Model file for the job. Use its own axes, mm. Give positions to 0.01 mm unless a question says otherwise; leave off trailing zeros. Order: outer loops, then holes, each group sorted by start corner. A loop starts at its lowest first (then second) coordinate and runs counter-clockwise, first axis right, second up. Notation, with made-up numbers: (50.25, 66) -> (95.25, 66) arc R8 ccw to (95.25, 70) -> close; hole circle Ø4 at (9, 80). An arc over 180 degrees is marked (long way). Use CSV: the item, a comma, the result in double quotes. Start each with the question number.
1. Cut at B-B on y = 6. List the corners of the cut face in (x, z).
2. Wall check: line 1 (X direction, y = 93, z = 12.5); line 2 (X direction, y = 21, z = -18); line 3 (Y direction, x = 22, z = -18). Give the ranges that are in metal, low to high. Write a range as from..to.
3. Pull direction X, two halves, no side cores. Call faces 1 (the cylindrical face through (142.94, 50.56, 23.72)), 2 (the cylindrical face through (-51.2, 50.56, -20.42)), 3 (the flat face through (45, 0, 1)): released by +X, released by -X, zero draft, split by the parting line, or undercut.
4. Cut at A-A on x = 107. List the corners of the cut face in (y, z).
```python
from build123d import *

# Parameters (mm, degrees)
ESBO_O1_W                = 200
ESBO_O1_H                = 50
RESSALTO_EXTRUS_O1_DEPTH = 100
FILETE9_R                = 10


with BuildPart() as part:
    # Esboço1 → Ressalto-extrusão1 (new body)
    with BuildSketch(Plane(origin=(0, 0, 0), x_dir=(1, 0, 0), z_dir=(0, 1, 0))):
        with Locations((45.947958133, -1.570526198)):
            Rectangle(ESBO_O1_W, ESBO_O1_H)
    extrude(amount=RESSALTO_EXTRUS_O1_DEPTH)

    # Filete9
    filete9_edges = [part.edges().sort_by_distance(p)[0] for p in [
        (145.947958133, 100, 1.570526198),
        (45.947958133, 100, -23.429473802),
        (-54.052041867, 100, 1.570526198),
        (45.947958133, 0, -23.429473802),
        (145.947958133, 0, 1.570526198),
        (45.947958133, 0, 26.570526198),
        (-54.052041867, 0, 1.570526198),
        (45.947958133, 100, 26.570526198),
        (-54.052041867, 50, -23.429473802),
        (145.947958133, 50, -23.429473802),
        (145.947958133, 50, 26.570526198),
        (-54.052041867, 50, 26.570526198),
    ]]
    fillet(filete9_edges, radius=FILETE9_R)


solid = part.part
```
Verdict:
1,outline,"(-53.22, -13.43) arc R9.17 ccw to (-44.05, -22.59) -> (135.95, -22.59) arc R9.17 ccw to (145.11, -13.43) -> (145.11, 16.57) arc R9.17 ccw to (135.95, 25.74) -> (-44.05, 25.74) arc R9.17 ccw to (-53.22, 16.57) -> close"
2,line 1,"-53.59..145.49"
2,line 2,"-52.95..144.84"
2,line 3,"1.11..98.89"
3,face 1,"released by +X"
3,face 2,"released by -X"
3,face 3,"zero draft"
4,outline,"(0, -13.43) arc R10 ccw to (10, -23.43) -> (90, -23.43) arc R10 ccw to (100, -13.43) -> (100, 16.57) arc R10 ccw to (90, 26.57) -> (10, 26.57) arc R10 ccw to (0, 16.57) -> close"
